```python
from build123d import *

# Parameters (mm, degrees)
F0_R     = 2.65
F1_DEPTH = 6
F3_DEPTH = 20
F4_R     = 3
F5_DEPTH = 25.4


with BuildPart() as f1:
    # F0 (on Right) → F1 (new body)
    with BuildSketch(Plane.YZ):
        with BuildLine():
            Line((-5.755054, 20), (-15.081208, 0))
            Line((-15.081208, 0), (0, 0))
            Line((0, 0), (15.081208, 0))
            Line((15.081208, 0), (5.755054, 20))
            ThreePointArc((5.755054, 20), (0, 23.666374), (-5.755054, 20))
        make_face()
        with Locations((0, 15)):
            Circle(F0_R, mode=Mode.SUBTRACT)
    extrude(amount=F1_DEPTH)

    # F2 (on Right) → F3 (join)
    with BuildSketch(Plane.YZ):
        Polygon((-13.813353, 2.718923), (-15.081208, 0), (15.081208, 0), (13.813353, 2.718923), align=None)
    extrude(amount=F3_DEPTH)

    # F4 (on Top) → F5 (cut)
    with BuildSketch(Plane.XY):
        with Locations((14, -8)):
            Circle(F4_R)
        with Locations((14, 8)):
            Circle(F4_R)
    extrude(amount=F5_DEPTH, mode=Mode.SUBTRACT)


solid = f1.part
```
Here's how the part is built. I have some questions about the finished solid (model axes, mm). A direction names the side the tool comes from. Coordinates: 2 decimals unless noted, no trailing zeros. Loops run counter-clockwise (first coordinate to the right, second up) from the corner with the lowest first, then second, coordinate; pieces in that order, holes last. Notation, with made-up numbers: M 78,37.25 L 86,37.25 A24 ccw 86,57.25 Z; hole C -34,69 d11. An arc over 180 degrees is marked long. One line per item, written item: value.
1. Thinking about a two-plate mould opening in X: for faces 3 (the cylindrical face through (11, 8, 1)), 4 (the cylindrical face through (2.958, 1.223, 12.649)), 5 (the flat face through (0, 0, 9)), which applies, +X half, -X half, draft (parallel to the pull), parting line (faces both ways), or undercut?
Geometry says:
face 3: undercut
face 4: draft
face 5: -X half
2. Will these pins go through, and if not, where does the flat tip stop? pin 1 Ø4 at (x, y) = (9.5, -0.5) entering from +Z; pin 2 Ø8 at (x, z) = (7.5, 6.5) entering from -Y; pin 3 Ø6.5 at (y, z) = (-5.5, 17.5) entering from +X.
Geometry says:
pin 1: stops at z = 2.72
pin 2: stops at y = -13.92
pin 3: stops at x = 6
3. Imagine slicing it at A-A (y = 0). List the corners of the cut face in (x, z) for me.
Geometry says:
outline: M 0,0 L 20,0 L 20,2.72 L 6,2.72 L 6,12.35 L 0,12.35 Z; M 0,17.65 L 6,17.65 L 6,23.67 L 0,23.67 Z
4. On a 3-axis mill with a long thin cutter (end or side, diameter ignored), from which of +Z, -Z, +X, -X, +Y, -Y can I reach the whole of each face in a straight line? I mean faces 1 (the flat face through (13, 0, 2.719)), 2 (the cylindrical face through (2.958, 0.101, 23.666)). Say none if no direction works.
Geometry says:
face 1: +Z, +X, +Y, -Y
face 2: +Z, +X, -X
5. Imagine slicing it at C-C (z = 15). List the corners of the cut face in (x, y) for me, and give its area (3 significant figures).
Geometry says:
outline: M 0,-8.09 L 6,-8.09 L 6,-2.65 L 0,-2.65 Z; M 0,2.65 L 6,2.65 L 6,8.09 L 0,8.09 Z
area: 65.2 mm2
6. Imagine slicing it at D-D (y = -10). List the corners of the cut face in (x, z) for me.
Geometry says:
outline: M 0,0 L 11.76,0 L 11.76,2.72 L 6,2.72 L 6,10.9 L 0,10.9 Z; M 16.24,0 L 20,0 L 20,2.72 L 16.24,2.72 Z
7. Please list where these lines run through material, in increasing order: probe 1 along X at (y, z) = (-8, 1.4); probe 2 along Y at (x, z) = (14, 1.8); probe 3 along Z at (x, y) = (11.5, -10.5).
Geometry says:
probe 1: x = 0 to 11, 17 to 20
probe 2: y = -14.24 to -11, -5 to 5, 11 to 14.24
probe 3: z = 0 to 2.72
8. Imagine slicing it at B-B (x = 14). List the corners of the cut face in (y, z) for me.
Geometry says:
outline: M -15.08,0 L -11,0 L -11,2.72 L -13.81,2.72 Z; M -5,0 L 5,0 L 5,2.72 L -5,2.72 Z; M 11,0 L 15.08,0 L 13.81,2.72 L 11,2.72 Z
